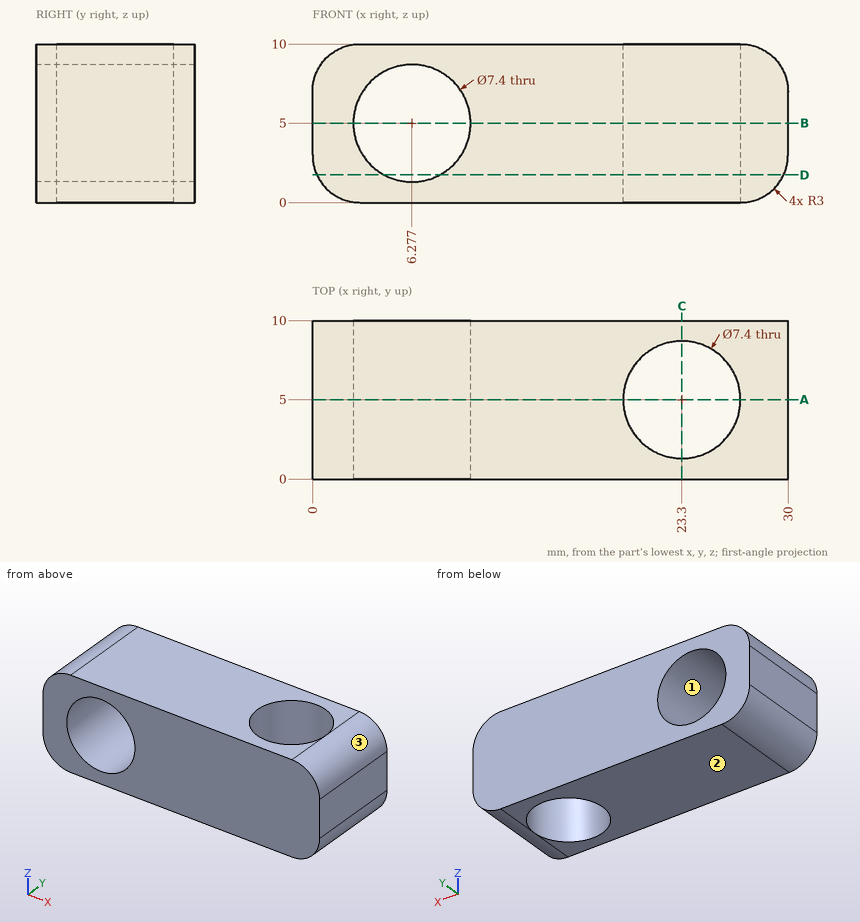
Study the drawing (mm; zero at the part's minimum x, y, z) and answer. Coordinates: 2 decimals unless noted, no trailing zeros. Write each loop counter-clockwise with the first axis right and the second up, starting at its lowest first coordinate (ties: lowest second). Pieces come first, ordered by that corner, then holes.
Q1. A cutting plane is placed at D-D, the plane z = 1.75. Give the vertices of the cut face in (x, y), then the cut area to 3 significant figures.
Q2. Find the intervals of material crossed by line 1 (Y direction, x = 23.5, z = 7.5) (1 decimal); line 2 (X direction, y = 2.5, z = 3) (1 decimal); line 3 (X direction, y = 2.25, z = 8.25) (1 decimal), in increasing order.
Q3. Determine the mould class of the marked faces 1, 2 and 3 for opening direction X: released by +X, released by -X, zero draft, split by the parting line, or undercut.
Q4. A cutting plane is placed at A-A, the plane y = 5. State how many separate pieces and enclosed holes the cut face has, then the cut area to 3 significant figures.
Q5. A cutting plane is placed at B-B, the plane z = 5. Give the vertices of the cut face in (x, y).
Q6. Each of these flat-tipped pins is pushed along its axis until it touches: pin 1 Ø1.5 at (y, z) = (3.5, 2) entering from -X; pin 2 Ø3 at (x, y) = (24, 3.5) entering from +Z. Where does it stop, or does it pass through?
Q7. A cutting plane is placed at C-C, the plane x = 23.3. Give the vertices of the cut face in (y, z).
Findings below:
1. outline: (0.27, 0) - (4.51, 0) - (4.51, 10) - (0.27, 10) - close; (8.05, 0) - (29.73, 0) - (29.73, 10) - (8.05, 10) - close; hole circle Ø7.4 at (23.3, 5)
1. area: 216 mm2
2. line 1: y = 0 to 1.3, 8.7 to 10
2. line 2: x = 0 to 3.2, 9.4 to 20.6, 26 to 30
2. line 3: x = 0.3 to 4.5, 8 to 20.8, 25.8 to 29.7
3. face 1: undercut
3. face 2: zero draft
3. face 3: released by +X
4. separate pieces: 2
4. enclosed holes: 1
4. area: 175 mm2
5. outline: (0, 0) - (2.58, 0) - (2.58, 10) - (0, 10) - close; (9.98, 0) - (30, 0) - (30, 10) - (9.98, 10) - close; hole circle Ø7.4 at (23.3, 5)
6. pin 1: stops at x = 0.01
6. pin 2: passes through
7. outline: (0, 0) - (1.3, 0) - (1.3, 10) - (0, 10) - close; (8.7, 0) - (10, 0) - (10, 10) - (8.7, 10) - close
